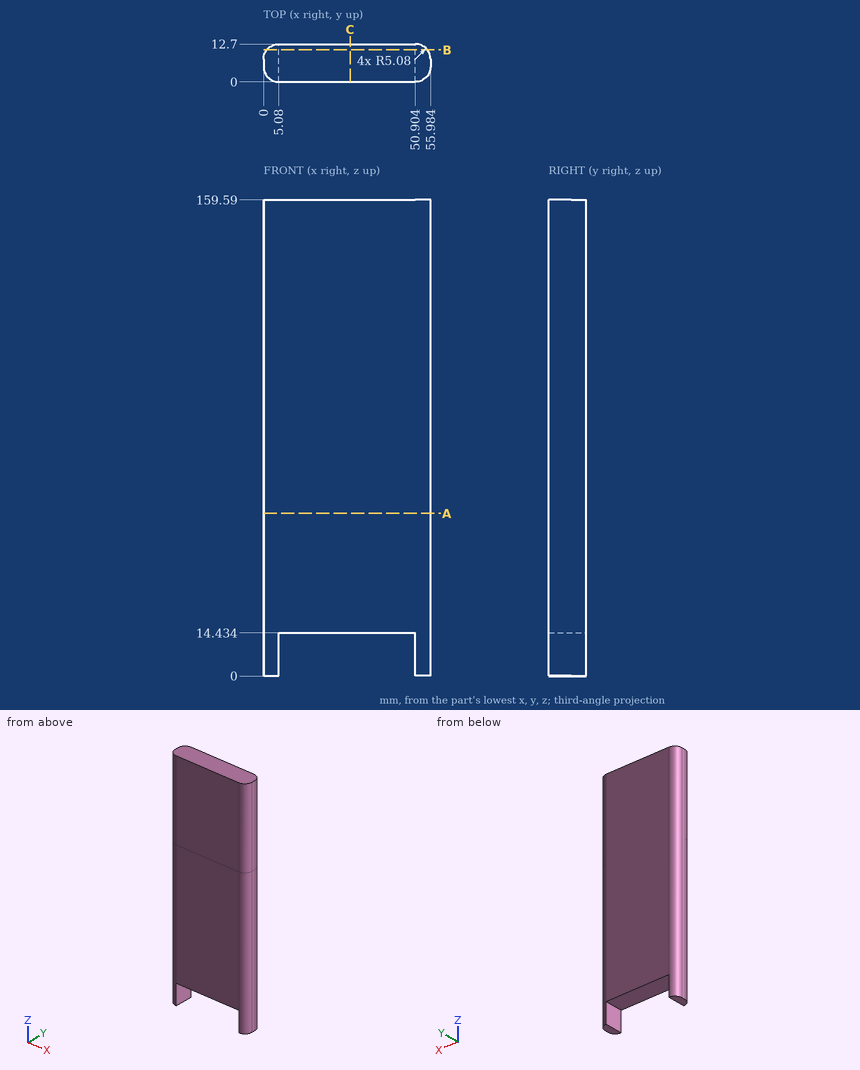
Print and shaded views of the part. All mm, measured from the part's lowest x, y and z. Round coordinates to 2 decimals unless told otherwise and drop trailing zeros. Write each loop counter-clockwise with the first axis right and the second up, starting at its lowest first coordinate (ties: lowest second). Pieces come first, ordered by that corner, then holes.
Item 1: Cut at B-B, the plane y = 10.75. Give the cut face in (x, z) (1 decimal), plus the area to 3 significant figures.
Results:
outline: (1.1, 0) - (5.1, 0) - (5.1, 14.4) - (50.9, 14.4) - (50.9, 0) - (54.9, 0) - (54.9, 159.6) - (1.1, 159.6) - close
area: 7,930 mm2
Item 2: Cut at A-A, the plane z = 54.5. Give the cut face in (x, y) (1 decimal).
Results:
outline: (0, 5.1) arc R5.1 ccw to (5.1, 0) - (50.9, 0) arc R5.1 ccw to (56, 5.1) - (56, 7.6) arc R5.1 ccw to (50.9, 12.7) - (5.1, 12.7) arc R5.1 ccw to (0, 7.6) - close
Item 3: Drop flat-ended pins along their axis: pin 1 Ø1 at (x, y) = (18, 7.5) entering from -Z (1 decimal); pin 2 Ø8 at (x, z) = (27, 30) entering from -Y. Give the stop position or say it passes through.
Results:
pin 1: stops at z = 14.4
pin 2: stops at y = 0
Item 4: Probe L1, parallel to Z at x = 32, y = 11 (1 decimal); L2, parallel to X at y = 8, z = 47 (1 decimal); L3, parallel to X at y = 10.5, z = 127 (1 decimal). List the from-to ranges inside material, lowest first.
Results:
L1: z = 14.4 to 159.6
L2: x = 0 to 56
L3: x = 0.9 to 55.1
Item 5: Cut at C-C, the plane x = 29. Give the cut face in (y, z) (1 decimal).
Results:
outline: (0, 14.4) - (12.7, 14.4) - (12.7, 159.6) - (0, 159.6) - close
